from build123d import *

# Parameters (mm, degrees)
SKETCH1_W           = 203.2
SKETCH1_H           = 101.6
BOSS_EXTRUDE1_DEPTH = 6.35
SKETCH2_W           = 6.35
SKETCH2_H           = 12.7
CUT_EXTRUDE1_DEPTH  = 6.35
SKETCH5_W           = 6.35
SKETCH5_H           = 6.35
CUT_EXTRUDE3_DEPTH  = 6.35
LPATTERN1_COUNT     = 15
LPATTERN1_PITCH     = 12.7
SKETCH6_W           = 6.35
SKETCH6_H           = 6.35
CUT_EXTRUDE4_DEPTH  = 6.35
SKETCH7_W           = 6.35
SKETCH7_H           = 6.35
CUT_EXTRUDE5_DEPTH  = 6.35
LPATTERN2_COUNT     = 7
LPATTERN2_PITCH     = 12.7
CUT_EXTRUDE6_DEPTH  = 6.35
SKETCH9_W           = 6.35
SKETCH9_H           = 6.35
CUT_EXTRUDE7_DEPTH  = 6.35
LPATTERN3_COUNT     = 3
LPATTERN3_PITCH     = 12.7
SKETCH10_W          = 25.9
SKETCH10_H          = 5
CUT_EXTRUDE8_DEPTH  = 6.35


with BuildPart() as part:
    # Sketch1 → Boss-Extrude1 (new body)
    with BuildSketch(Plane(origin=(0, 0, 0), x_dir=(0, 0, -1), z_dir=(1, 0, 0))):
        with Locations((101.6, 50.8)):
            Rectangle(SKETCH1_W, SKETCH1_H)
    extrude(amount=BOSS_EXTRUDE1_DEPTH)

    # Sketch2 → Cut-Extrude1 (cut)
    with BuildSketch(Plane.XZ):
        with Locations((3.175, -6.35)):
            Rectangle(SKETCH2_W, SKETCH2_H)
    extrude(amount=-CUT_EXTRUDE1_DEPTH, mode=Mode.SUBTRACT)

    # Sketch5 → Cut-Extrude3 (cut)
    with BuildSketch(Plane.XZ):
        with Locations((3.175, -22.225)):
            Rectangle(SKETCH5_W, SKETCH5_H)
    cut_extrude3 = extrude(amount=-CUT_EXTRUDE3_DEPTH, mode=Mode.SUBTRACT)

    # LPattern1: Cut-Extrude3 ×15
    with Locations(*[(0, 0, -i * LPATTERN1_PITCH) for i in range(1, LPATTERN1_COUNT)]):
        add(cut_extrude3, mode=Mode.SUBTRACT)

    # Sketch6 → Cut-Extrude4 (cut)
    with BuildSketch(Plane(origin=(0, 0, -203.2), x_dir=(-1, 0, 0), z_dir=(0, 0, -1))):
        with Locations((-3.175, 9.525)):
            Rectangle(SKETCH6_W, SKETCH6_H)
    extrude(amount=-CUT_EXTRUDE4_DEPTH, mode=Mode.SUBTRACT)

    # Sketch7 → Cut-Extrude5 (cut)
    with BuildSketch(Plane(origin=(0, 0, -203.2), x_dir=(-1, 0, 0), z_dir=(0, 0, -1))):
        with Locations((-3.175, 22.225)):
            Rectangle(SKETCH7_W, SKETCH7_H)
    cut_extrude5 = extrude(amount=-CUT_EXTRUDE5_DEPTH, mode=Mode.SUBTRACT)

    # LPattern2: Cut-Extrude5 ×7
    with Locations(*[(0, i * LPATTERN2_PITCH, 0) for i in range(1, LPATTERN2_COUNT)]):
        add(cut_extrude5, mode=Mode.SUBTRACT)

    # Sketch8 → Cut-Extrude6 (cut)
    with BuildSketch(Plane(origin=(6.35, 0, 0), x_dir=(0, 0, -1), z_dir=(1, 0, 0))):
        Polygon((0, 101.6), (50.8, 101.6), (0, 50.8), align=None)
    extrude(amount=-CUT_EXTRUDE6_DEPTH, mode=Mode.SUBTRACT)

    # Sketch9 → Cut-Extrude7 (cut)
    with BuildSketch(Plane.XY):
        with Locations((3.175, 15.875)):
            Rectangle(SKETCH9_W, SKETCH9_H)
    cut_extrude7 = extrude(amount=-CUT_EXTRUDE7_DEPTH, mode=Mode.SUBTRACT)

    # LPattern3: Cut-Extrude7 ×3
    with Locations(*[(0, i * LPATTERN3_PITCH, 0) for i in range(1, LPATTERN3_COUNT)]):
        add(cut_extrude7, mode=Mode.SUBTRACT)

    # Sketch10 → Cut-Extrude8 (cut)
    with BuildSketch(Plane(origin=(6.35, 0, 0), x_dir=(0, 0, -1), z_dir=(1, 0, 0))):
        with Locations((152.15, 21.55)):
            Rectangle(SKETCH10_W, SKETCH10_H)
    extrude(amount=-CUT_EXTRUDE8_DEPTH, mode=Mode.SUBTRACT)


solid = part.part
Can you work these out from the model? Positions are in its coordinate system, mm. A direction names the side the tool comes from. Give positions to 0.01 mm unless a question says otherwise; leave off trailing zeros. Order: outer loops, then holes, each group sorted by start corner. A loop starts at its lowest first (then second) coordinate and runs counter-clockwise, first axis right, second up. Notation, with made-up numbers: M 41,1 L 64,1 A20 ccw 64,34 Z; hole C -38.5,-25.75 d4. An arc over 180 degrees is marked long. Use a Markdown table: item, result. Add a question column.
Item 1: Suppose I cut it at A-A (z = -149). List the corners of the cut face in (x, y) for me, then the cut area to 3 significant figures.
Item 2: For faces 5 (the flat face through (3, 12.7, -200)), 6 (the flat face through (3, 6.35, -111)), 7 (the flat face through (3, 76.2, -200)), which set-ups out of +Z, -Z, +X, -X, +Y, -Y let a thin tool reach every point of the face, with its end or its side?
Item 3: If I drill on L1, parallel to Y at x = 3.5, z = -152; L2, parallel to Y at x = 5.25, z = -186; L3, parallel to Z at x = 4.25, y = 47.5, over which ranges is the centre line in solid material (lowest first)? Write a range as [from, to].
Item 4: Suppose I cut it at C-C (y = 72). List the corners of the cut face in (x, z) for me.
Item 5: Suppose I cut it at B-B (y = 46.5). List the corners of the cut face in (x, z) for me, then the cut area to 3 significant figures.
Item 6: Will these pins go through, and if not, where does the flat tip stop? pin 1 (3 mm diameter, centred on x = 3, y = 3, fed in from -Z); pin 2 (3 mm diameter, centred on x = 4.5, z = -36, fed in from -Y); pin 3 (1.9 mm diameter, centred on x = 3, y = 4.5, fed in from +Z).
Item 7: We'd pull the mould along Z, two halves only. Please class faces 1 (the flat face through (3, 31.75, -200)), 2 (the flat face through (3, 16, -203.2)), 3 (the flat face through (3, 3, -95.25)), 4 (the flat face through (3, 35, 0)): +Z half, -Z half, draft (parallel to the pull), parting line (faces both ways), or undercut.
Answer sheet:
| question | item | result |
|---|---|---|
| 1 | outline | M 0,6.35 L 6.35,6.35 L 6.35,19.05 L 0,19.05 Z; M 0,24.05 L 6.35,24.05 L 6.35,101.6 L 0,101.6 Z |
| 1 | area | 573 mm² |
| 2 | face 5 | -Z, +X, -X, -Y |
| 2 | face 6 | +X, -X, -Y |
| 2 | face 7 | -Z, +X, -X |
| 3 | L1 | y = [6.35, 19.05], [24.05, 101.6] |
| 3 | L2 | y = [6.35, 101.6] |
| 3 | L3 | z = [-196.85, 0] |
| 4 | outline | M 0,-196.85 L 6.35,-196.85 L 6.35,-21.2 L 0,-21.2 Z |
| 5 | outline | M 0,-196.85 L 6.35,-196.85 L 6.35,0 L 0,0 Z |
| 5 | area | 1,250 mm² |
| 6 | pin 1 | stops at z = -196.85 |
| 6 | pin 2 | stops at y = 6.35 |
| 6 | pin 3 | stops at z = -12.7 |
| 7 | face 1 | draft |
| 7 | face 2 | -Z half |
| 7 | face 3 | undercut |
| 7 | face 4 | +Z half |
